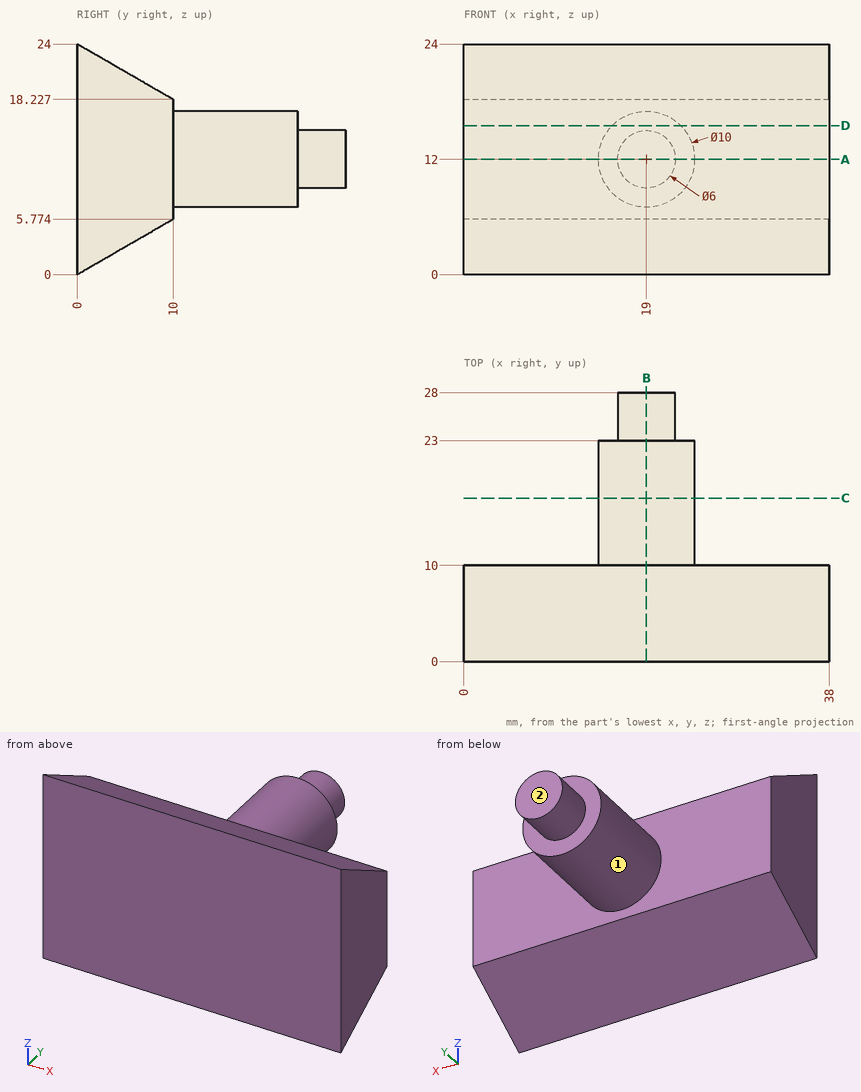
Job drawing, mm, ordinate dimensions from the low corner. One solid piece. A direction names the side the tool comes from. Round coordinates to 2 decimals unless told otherwise and drop trailing zeros. Write each loop counter-clockwise with the first axis right and the second up, starting at its lowest first coordinate (ties: lowest second). Pieces come first, ordered by that corner, then holes.
1) 3-axis set-ups, long thin cutter, end or side, ignore diameter. For the marked faces 1 and 2: which of +Z, -Z, +X, -X, +Y, -Y reach the whole face in a straight line?
2) Band-saw the part on C-C, the plane y = 17. List the corners of the cut face in (x, z).
3) Band-saw the part on D-D, the plane z = 15.5. List the corners of the cut face in (x, y).
4) Band-saw the part on B-B, the plane x = 19. List the corners of the cut face in (y, z).
5) Pin check, flat tips, straight feed: pin 1 (10 mm diameter, centred on x = 8.5, z = 6, fed in from +Y); pin 2 (8 mm diameter, centred on x = 10.5, y = 17, fed in from -Z); pin 3 (5 mm diameter, centred on x = 17.5, y = 4.5, fed in from -Z) (1 decimal). Stop position of each tip, or through.
6) Drill centre lines: probe 1 along Y at (x, z) = (33.5, 6); probe 2 along Z at (x, y) = (23, 12.5); probe 3 along Z at (x, y) = (4.5, 5.25). Where is each one in solid material? Low to high.
7) Band-saw the part on A-A, the plane z = 12. List the corners of the cut face in (x, y), and give its area (3 significant figures).
Ans:
1. face 1: +Y
1. face 2: +Z, -Z, +X, -X, +Y
2. outline: circle Ø10 at (19, 12)
3. outline: (0, 0) - (38, 0) - (38, 10) - (22.57, 10) - (22.57, 23) - (15.43, 23) - (15.43, 10) - (0, 10) - close
4. outline: (0, 0) - (10, 5.77) - (10, 7) - (23, 7) - (23, 9) - (28, 9) - (28, 15) - (23, 15) - (23, 17) - (10, 17) - (10, 18.23) - (0, 24) - close
5. pin 1: stops at y = 10
5. pin 2: stops at z = 9.82
5. pin 3: stops at z = 1.2
6. probe 1: y = 0 to 10
6. probe 2: z = 9 to 15
6. probe 3: z = 3.03 to 20.97
7. outline: (0, 0) - (38, 0) - (38, 10) - (24, 10) - (24, 23) - (22, 23) - (22, 28) - (16, 28) - (16, 23) - (14, 23) - (14, 10) - (0, 10) - close
7. area: 540 mm2
